CAD build for the part. Positions are in the model's coordinates, mm. A direction names the side the tool comes from. Coordinates: 2 decimals unless noted, no trailing zeros. Loops run counter-clockwise (first coordinate to the right, second up) from the corner with the lowest first, then second, coordinate; pieces in that order, holes last. Notation, with made-up numbers: (8, 24.5) -> (25, 24.5) arc R32 cw to (25, 58.5) -> close; hole circle Ø9 at (47.5, 8). An arc over 180 degrees is marked (long way). Answer as CSV lines item,"result". Start each with the question number.
```python
from build123d import *

# Parameters (mm, degrees)
SKETCH1_R           = 24.5
SKETCH1_R_2         = 18.5
BOSS_EXTRUDE1_DEPTH = 4.5
SKETCH2_R           = 24.5
BOSS_EXTRUDE2_DEPTH = 2
SKETCH3_R           = 1.5
CUT_EXTRUDE1_DEPTH  = 36.252659474


with BuildPart() as part:
    # Sketch1 → Boss-Extrude1 (new body)
    with BuildSketch(Plane(origin=(0, 0, 0), x_dir=(1, 0, 0), z_dir=(0, 1, 0))):
        with Locations(Location((0, 0, 0), (0, 0, 270))):
            Circle(SKETCH1_R)
        with Locations(Location((0, 0, 0), (0, 0, 270))):
            Circle(SKETCH1_R_2, mode=Mode.SUBTRACT)
    extrude(amount=BOSS_EXTRUDE1_DEPTH)

    # Sketch2 → Boss-Extrude2 (add)
    with BuildSketch(Plane(origin=(0, 4.5, 0), x_dir=(1, 0, 0), z_dir=(0, 1, 0))):
        with Locations(Location((0, 0, 0), (0, 0, 270))):
            Circle(SKETCH2_R)
    extrude(amount=BOSS_EXTRUDE2_DEPTH)

    # Sketch3 → Cut-Extrude1 (cut, through all)
    with BuildSketch(Plane.XZ):
        with Locations(Location((0, -21.25, 0), (0, 0, 270))):
            Circle(SKETCH3_R)
        with Locations(Location((0, 21.25, 0), (0, 0, 270))):
            Circle(SKETCH3_R)
    extrude(amount=-CUT_EXTRUDE1_DEPTH, mode=Mode.SUBTRACT)


solid = part.part
```
Q1. Saw through at A-A (x = 0). List the corners of the cut face in (y, z), and give its area (3 significant figures).
Q2. Probe probe 1 along X at (y, z) = (1.6, 0); probe 2 along Y at (x, z) = (9.5, 5); probe 3 along X at (y, z) = (3.25, 10). List the from-to ranges inside material, lowest first. Write a range as from..to.
Q3. Pin check, flat tips, straight feed: pin 1 Ø2 at (x, y) = (-4.5, 1) entering from +Z; pin 2 Ø4 at (x, z) = (7.5, -4) entering from -Y; pin 3 Ø2.5 at (x, z) = (0, -21.25) entering from -Y. Stop position of each tip, or through.
Q4. Saw through at D-D (z = 0). List the corners of the cut face in (x, y), and give its area (3 significant figures).
Q5. Saw through at B-B (z = -21.25). List the corners of the cut face in (x, y), and give its area (3 significant figures).
Q6. Saw through at C-C (y = 5.25). List the corners of the cut face in (x, z), and give its area (3 significant figures).
Q7. Which spindle directions (+Z, -Z, +X, -X, +Y, -Y) get a long thin tool onto all of the face, cutting with end or side? Do faces 1 (the flat face through (0, 6.5, 0)), 2 (the flat face through (0, 4.5, 0)). Say none if no direction does.
Q8. Two-plate mould, pull along Z, no slides. Class faces 3 (the cylindrical face through (-7.086, 2.218, 17.089)), 4 (the flat face through (16.4, 0, 9)), 5 (the cylindrical face through (7.36, 3.2, 23.37)): pulls with the +Z half, pulls with the -Z half, needs draft (parallel to the pull), parting line crosses it, or undercut.
Ans:
1,outline,"(0, -24.5) -> (6.5, -24.5) -> (6.5, -22.75) -> (0, -22.75) -> close; (0, -19.75) -> (6.5, -19.75) -> (6.5, 19.75) -> (0, 19.75) -> (0, 18.5) -> (4.5, 18.5) -> (4.5, -18.5) -> (0, -18.5) -> close; (0, 22.75) -> (6.5, 22.75) -> (6.5, 24.5) -> (0, 24.5) -> close"
1,area,"113 mm²"
2,probe 1,"x = -24.5..-18.5, 18.5..24.5"
2,probe 2,"y = 4.5..6.5"
2,probe 3,"x = -22.37..-15.56, 15.56..22.37"
3,pin 1,"stops at z = 24.25"
3,pin 2,"stops at y = 4.5"
3,pin 3,"passes through"
4,outline,"(-24.5, 0) -> (-18.5, 0) -> (-18.5, 4.5) -> (18.5, 4.5) -> (18.5, 0) -> (24.5, 0) -> (24.5, 6.5) -> (-24.5, 6.5) -> close"
4,area,"152 mm²"
5,outline,"(-12.19, 0) -> (-1.5, 0) -> (-1.5, 6.5) -> (-12.19, 6.5) -> close; (1.5, 0) -> (12.19, 0) -> (12.19, 6.5) -> (1.5, 6.5) -> close"
5,area,"139 mm²"
6,outline,"circle Ø49 at (0, 0); hole circle Ø3 at (0, -21.25); hole circle Ø3 at (0, 21.25)"
6,area,"1,870 mm²"
7,face 1,"+Z, -Z, +X, -X, +Y"
7,face 2,"-Y"
8,face 3,"undercut"
8,face 4,"needs draft"
8,face 5,"parting line crosses it"
